from build123d import *

# Parameters (mm, degrees)
SKETCH021_W     = 36
SKETCH021_H     = 36
PAD006_DEPTH    = 3
SKETCH022_W     = 43.5
SKETCH022_H     = 43.5
PAD007_DEPTH    = 8.75
POCKET014_DEPTH = 100
POCKET015_DEPTH = 100
SKETCH025_W     = 28
SKETCH025_H     = 28
POCKET016_DEPTH = 7.75
SKETCH026_R     = 4.5
POCKET017_DEPTH = 3
SKETCH030_R     = 2.6
POCKET021_DEPTH = 5
CHAMFER003_SIZE = 1.75


with BuildPart() as part:
    # Sketch021 (on Face1 of ShapeBinder003) → Pad006 (new body)
    with BuildSketch(Plane(origin=(0, 0, 0), x_dir=(1, 0, 0), z_dir=(0, 0, -1))):
        with Locations((124, -211)):
            Rectangle(SKETCH021_W, SKETCH021_H)
    extrude(amount=PAD006_DEPTH)

    # Sketch022 (on Face6 of Pad006) → Pad007 (join)
    with BuildSketch(Plane(origin=(0, 0, -3), x_dir=(1, 0, 0), z_dir=(0, 0, -1))):
        with Locations((124, -211)):
            Rectangle(SKETCH022_W, SKETCH022_H)
    extrude(amount=PAD007_DEPTH)

    # Sketch023 (on Face1 of Pad007) → Pocket014 (cut)
    with BuildSketch(Plane.XZ.offset(-189.25)):
        Polygon((106, -3), (102.25, -9.75), (102.25, -3), align=None)
        Polygon((142, -3), (145.75, -9.75), (145.75, -3), align=None)
    extrude(amount=-POCKET014_DEPTH, mode=Mode.SUBTRACT)

    # Sketch024 (on Face7 of Pocket014) → Pocket015 (cut)
    with BuildSketch(Plane(origin=(102.25, 0, 0), x_dir=(0, -1, 0), z_dir=(-1, 0, 0))):
        Polygon((-229, -3), (-232.75, -9.75), (-232.75, -3), align=None)
        Polygon((-193, -3), (-189.25, -3), (-189.25, -9.75), align=None)
    extrude(amount=-POCKET015_DEPTH, mode=Mode.SUBTRACT)

    # Sketch025 (on Face4 of Pocket015) → Pocket016 (cut)
    with BuildSketch(Plane(origin=(0, 0, -11.75), x_dir=(1, 0, 0), z_dir=(0, 0, -1))):
        with Locations((124, -211)):
            Rectangle(SKETCH025_W, SKETCH025_H)
    extrude(amount=-POCKET016_DEPTH, mode=Mode.SUBTRACT)

    # Sketch026 (on Face18 of Pocket016) → Pocket017 (cut)
    with BuildSketch(Plane(origin=(0, 0, -4), x_dir=(1, 0, 0), z_dir=(0, 0, -1))):
        with Locations((116.5, -218.5)):
            Circle(SKETCH026_R)
        with Locations((131.5, -203.5)):
            Circle(SKETCH026_R)
    extrude(amount=-POCKET017_DEPTH, mode=Mode.SUBTRACT)

    # Sketch030 (on Face18 of Pocket017) → Pocket021 (cut)
    with BuildSketch(Plane(origin=(0, 0, -4), x_dir=(1, 0, 0), z_dir=(0, 0, -1))):
        with Locations((116.5, -218.5)):
            Circle(SKETCH030_R)
        with Locations((131.5, -203.5)):
            Circle(SKETCH030_R)
    extrude(amount=-POCKET021_DEPTH, mode=Mode.SUBTRACT)

    # Chamfer003
    chamfer003_edges = [part.edges().sort_by_distance(p)[0] for p in [
        (112, 218.5, -1),
        (127, 203.5, -1),
    ]]
    chamfer(chamfer003_edges, length=CHAMFER003_SIZE)


solid = part.part
The model under review builds one solid part; all positions refer to its coordinate system, in mm. A direction names the side the tool comes from. Round coordinates to 2 decimals unless told otherwise and drop trailing zeros. Order: outer loops, then holes, each group sorted by start corner. A loop starts at its lowest first (then second) coordinate and runs counter-clockwise, first axis right, second up. Notation, with made-up numbers: (26, -2) - (42, -2) arc R16 cw to (42, 28) - close; hole circle Ø3 at (63.25, 56). An arc over 180 degrees is marked (long way). Use one line per item in the form item = value.
Q1. Clearance check with flat-ended pins moving along their axes: P1, Ø6, axis at y = 208.5, z = -6, coming from the -X side; P2, Ø2, axis at y = 218, z = -3.5, coming from the +X side; P3, Ø10.5, axis at x = 131.5, y = 203.5, coming from the +Z side; P4, Ø5, axis at x = 109, z = -5, coming from the +Y side. State where each tip first meets the part, or that it passes through.
Response values:
P1 = 102.67
P2 = 142.83
P3 = 0
P4 = 231.5
Q2. To check wall thickness, follow line 1 (Y direction, x = 116.5, z = -3); line 2 (Y direction, x = 131.5, z = -0.55); line 3 (X direction, y = 203.5, z = -0.5). State the ranges of each line that lie inside material, in increasing order.
Response values:
line_1 = 193 to 214, 223 to 229
line_2 = 193 to 200.9, 206.1 to 229
line_3 = 106 to 128.9, 134.1 to 142
Q3. Add section A-A on z = -5.25. Give the boundary of the cut face in (x, y).
Response values:
outline = (104.75, 191.75) - (143.25, 191.75) - (143.25, 230.25) - (104.75, 230.25) - close; hole (110, 197) - (138, 197) - (138, 225) - (110, 225) - close
Q4. Add section C-C on x = 116.5. Give the boundary of the cut face in (y, z), then the cut area to 3 significant figures.
Response values:
outline = (189.25, -11.75) - (197, -11.75) - (197, -4) - (214, -4) - (214, -2.75) - (215.75, -1) - (215.9, -1) - (215.9, 0) - (193, 0) - (193, -3) - (189.25, -9.75) - close; (221.1, -1) - (221.25, -1) - (223, -2.75) - (223, -4) - (225, -4) - (225, -11.75) - (232.75, -11.75) - (232.75, -9.75) - (229, -3) - (229, 0) - (221.1, 0) - close
area = 217 mm^2
Q5. Mouldability with a two-part tool opening along Y and no side actions: class faces 4 (the flat face through (124, 232.75, -11)), 5 (the flat face through (102.25, 211, -11)), 6 (the flat face through (138, 211, -8)) as pulls with the +Y half, pulls with the -Y half, needs draft (parallel to the pull), parting line crosses it, or undercut.
Response values:
face_4 = pulls with the +Y half
face_5 = needs draft
face_6 = undercut
Q6. Add section D-D on z = -2. Give the boundary of the cut face in (x, y), then the cut area to 3 significant figures.
Response values:
outline = (106, 193) - (142, 193) - (142, 229) - (106, 229) - close; hole circle Ø7.5 at (116.5, 218.5); hole circle Ø7.5 at (131.5, 203.5)
area = 1,210 mm^2
Q7. Tool access review of faces 1 (the flat face through (110, 211, -8)), 2 (the flat face through (124, 189.25, -11)), 3 (the flat face through (142, 211, -1)): name each direction out of +Z, -Z, +X, -X, +Y, -Y from which nothing blocks a thin tool from reaching the whole face with its end or side.
Response values:
face_1 = -Z
face_2 = +Z, -Z, +X, -X, -Y
face_3 = +Z, +X, +Y, -Y
Q8. Add section B-B on y = 203.5. Give the boundary of the cut face in (x, z).
Response values:
outline = (102.25, -11.75) - (110, -11.75) - (110, -4) - (127, -4) - (127, -2.75) - (128.75, -1) - (128.9, -1) - (128.9, 0) - (106, 0) - (106, -3) - (102.25, -9.75) - close; (134.1, -1) - (134.25, -1) - (136, -2.75) - (136, -4) - (138, -4) - (138, -11.75) - (145.75, -11.75) - (145.75, -9.75) - (142, -3) - (142, 0) - (134.1, 0) - close
